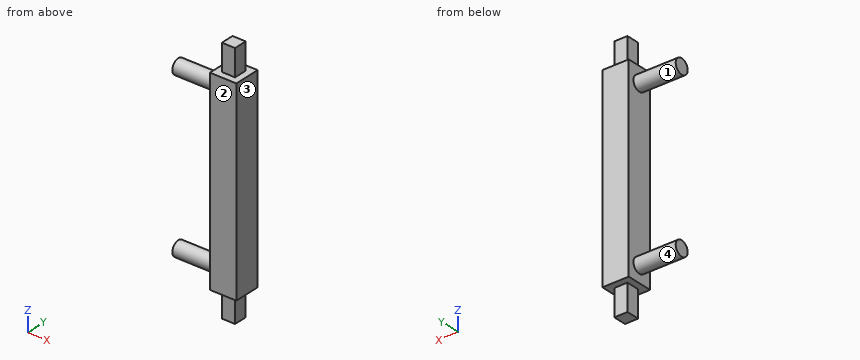
```python
from build123d import *

# Parameters (mm, degrees)
SKETCH1_W           = 5
SKETCH1_H           = 5
BOSS_EXTRUDE1_DEPTH = 37
SKETCH2_W           = 2.5
SKETCH2_H           = 2.5
BOSS_EXTRUDE2_DEPTH = 5
SKETCH3_W           = 2.5
SKETCH3_H           = 2.5
BOSS_EXTRUDE3_DEPTH = 5
SKETCH4_R           = 1.4
BOSS_EXTRUDE4_DEPTH = 8


with BuildPart() as part:
    # Sketch1 → Boss-Extrude1 (new body)
    with BuildSketch(Plane.XY):
        with Locations((2.5, 2.5)):
            Rectangle(SKETCH1_W, SKETCH1_H)
    extrude(amount=BOSS_EXTRUDE1_DEPTH)

    # Sketch2 → Boss-Extrude2 (add)
    with BuildSketch(Plane.XY.offset(37)):
        with Locations((2.5, 2.5)):
            Rectangle(SKETCH2_W, SKETCH2_H)
    extrude(amount=BOSS_EXTRUDE2_DEPTH)

    # Sketch3 → Boss-Extrude3 (add)
    with BuildSketch(Plane(origin=(0, 0, 0), x_dir=(-1, 0, 0), z_dir=(0, 0, -1))):
        with Locations((-2.5, 2.5)):
            Rectangle(SKETCH3_W, SKETCH3_H)
    extrude(amount=BOSS_EXTRUDE3_DEPTH)

    # Sketch4 → Boss-Extrude4 (add)
    with BuildSketch(Plane.ZY):
        with Locations(Location((3, 2.5, 0), (0, 0, 180))):
            Circle(SKETCH4_R)
        with Locations(Location((34, 2.5, 0), (0, 0, 180))):
            Circle(SKETCH4_R)
    extrude(amount=BOSS_EXTRUDE4_DEPTH)


solid = part.part
```
Geometry check sheet. Reference: the model listing, model coordinates, mm. Face numbers are marked on the shaded views. A direction names the side the tool comes from. Round coordinates to 2 decimals unless told otherwise and drop trailing zeros. Loops run counter-clockwise (first coordinate to the right, second up) from the corner with the lowest first, then second, coordinate; pieces in that order, holes last. Notation, with made-up numbers: (-11.75, 31.25) - (20.25, 31.25) arc R17 cw to (20.25, 63.25) - close; hole circle Ø3 at (25.5, 12.5). An arc over 180 degrees is marked (long way). Write each question's results on one line, items separated by ' | '. Start each with the question number.
Q1. Access from +Z, -Z, +X, -X, +Y, -Y to the whole of each face (thin tool, end or side, straight path). Record for the marked faces 1 and 2.
Q2. Release check for a two-part mould opening along Z. For the marked faces 3 and 4 record: +Z half, -Z half, draft (parallel to the pull), parting line (faces both ways), or undercut.
Q3. Cross-section at B-B on x = -5.25. Enter the section's corners in (y, z).
Q4. Gauge pin test, flat ends, axial feed: P1, Ø0.8, axis at x = 3, z = -1.5, coming from the -Y side; P2, Ø2, axis at x = -4, y = 2, coming from the +Z side; P3, Ø2.5, axis at y = 2, z = 27.5, coming from the -X side. Record the tip position at first contact, or that the pin passes through.
Q5. Cross-section at C-C on z = 3. Enter the section's corners in (x, y).
Q6. Cross-section at A-A on y = 2.5. Enter the section's corners in (x, z), and give its area (3 significant figures).
Q7. Cross-section at D-D on x = 2.5. Enter the section's corners in (y, z), and give its area (3 significant figures).
Q8. Thickness scan on line 1 (X direction, y = 0.95, z = 11); line 2 (Z direction, x = -2.75, y = 1.45); line 3 (Z direction, x = -3, y = 2.1). Record the ranges inside material, lowest first. Write a range as [from, to].
Answers below:
1) face 1: -X | face 2: +Z, -Z, +X, -X, -Y
2) face 3: draft | face 4: undercut
3) outline: circle Ø2.8 at (2.5, 3); circle Ø2.8 at (2.5, 34)
4) P1: stops at y = 1.25 | P2: stops at z = 35.4 | P3: stops at x = 0
5) outline: (-8, 1.1) - (0, 1.1) - (0, 0) - (5, 0) - (5, 5) - (0, 5) - (0, 3.9) - (-8, 3.9) - close
6) outline: (-8, 1.6) - (0, 1.6) - (0, 0) - (1.25, 0) - (1.25, -5) - (3.75, -5) - (3.75, 0) - (5, 0) - (5, 37) - (3.75, 37) - (3.75, 42) - (1.25, 42) - (1.25, 37) - (0, 37) - (0, 35.4) - (-8, 35.4) - (-8, 32.6) - (0, 32.6) - (0, 4.4) - (-8, 4.4) - close | area: 255 mm²
7) outline: (0, 0) - (1.25, 0) - (1.25, -5) - (3.75, -5) - (3.75, 0) - (5, 0) - (5, 37) - (3.75, 37) - (3.75, 42) - (1.25, 42) - (1.25, 37) - (0, 37) - close | area: 210 mm²
8) line 1: x = [0, 5] | line 2: z = [2.07, 3.93], [33.07, 34.93] | line 3: z = [1.66, 4.34], [32.66, 35.34]
